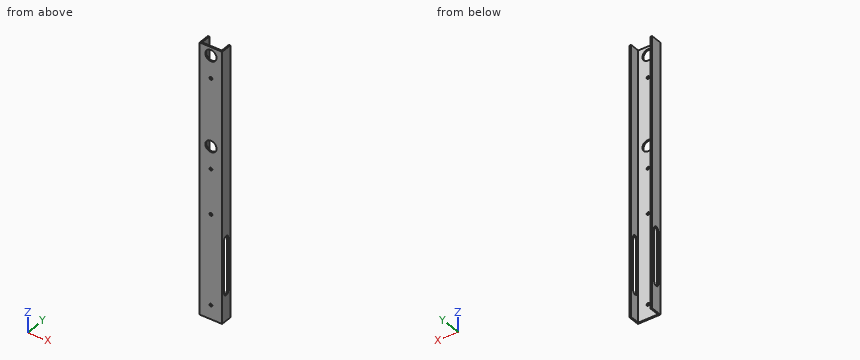
from build123d import *

# Parameters (mm, degrees)
BOSS_EXTRUDE1_DEPTH = 609.6
CUT_EXTRUDE1_REACH  = 5.175
SKETCH2_R           = 12.7
SKETCH2_R_2         = 3.175
CUT_EXTRUDE2_REACH  = 5.175
SKETCH3_R           = 3.175
CUT_EXTRUDE3_DEPTH  = 51.8


with BuildPart() as part:
    # Sketch1 → Boss-Extrude1 (new body)
    with BuildSketch(Plane.XY):
        Polygon((47.625, 3.175), (47.625, 25.4), (50.8, 25.4), (50.8, 0), (0, 0), (0, 25.4), (3.175, 25.4), (3.175, 3.175), align=None)
    extrude(amount=BOSS_EXTRUDE1_DEPTH)

    # Sketch2 → Cut-Extrude1 (cut, up to next)
    with BuildSketch(Plane(origin=(0, 3.175, 0), x_dir=(1, 0, 0), z_dir=(0, 1, 0)), mode=Mode.PRIVATE) as cut_extrude1_sk1:
        with Locations((25.4, -590.55)):
            Circle(SKETCH2_R)
    cut_extrude1_tool1 = extrude(cut_extrude1_sk1.sketch, amount=-CUT_EXTRUDE1_REACH, mode=Mode.PRIVATE) & part.part
    add(cut_extrude1_tool1.solids().sort_by_distance((25.4, 3.175, 590.55))[0], mode=Mode.SUBTRACT)
    # Sketch2 → Cut-Extrude1 (cut, up to next)
    with BuildSketch(Plane(origin=(0, 3.175, 0), x_dir=(1, 0, 0), z_dir=(0, 1, 0)), mode=Mode.PRIVATE) as cut_extrude1_sk2:
        with Locations((25.4, -387.35)):
            Circle(SKETCH2_R)
    cut_extrude1_tool2 = extrude(cut_extrude1_sk2.sketch, amount=-CUT_EXTRUDE1_REACH, mode=Mode.PRIVATE) & part.part
    add(cut_extrude1_tool2.solids().sort_by_distance((25.4, 3.175, 387.35))[0], mode=Mode.SUBTRACT)
    # Sketch2 → Cut-Extrude1 (cut, up to next)
    with BuildSketch(Plane(origin=(0, 3.175, 0), x_dir=(1, 0, 0), z_dir=(0, 1, 0)), mode=Mode.PRIVATE) as cut_extrude1_sk3:
        with Locations((25.4, -539.75)):
            Circle(SKETCH2_R_2)
    cut_extrude1_tool3 = extrude(cut_extrude1_sk3.sketch, amount=-CUT_EXTRUDE1_REACH, mode=Mode.PRIVATE) & part.part
    add(cut_extrude1_tool3.solids().sort_by_distance((25.4, 3.175, 539.75))[0], mode=Mode.SUBTRACT)
    # Sketch2 → Cut-Extrude1 (cut, up to next)
    with BuildSketch(Plane(origin=(0, 3.175, 0), x_dir=(1, 0, 0), z_dir=(0, 1, 0)), mode=Mode.PRIVATE) as cut_extrude1_sk4:
        with Locations((25.4, -336.55)):
            Circle(SKETCH2_R_2)
    cut_extrude1_tool4 = extrude(cut_extrude1_sk4.sketch, amount=-CUT_EXTRUDE1_REACH, mode=Mode.PRIVATE) & part.part
    add(cut_extrude1_tool4.solids().sort_by_distance((25.4, 3.175, 336.55))[0], mode=Mode.SUBTRACT)

    # Sketch3 → Cut-Extrude2 (cut, up to next)
    with BuildSketch(Plane(origin=(0, 3.175, 0), x_dir=(1, 0, 0), z_dir=(0, 1, 0)), mode=Mode.PRIVATE) as cut_extrude2_sk1:
        with Locations((25.4, -234.95)):
            Circle(SKETCH3_R)
    cut_extrude2_tool1 = extrude(cut_extrude2_sk1.sketch, amount=-CUT_EXTRUDE2_REACH, mode=Mode.PRIVATE) & part.part
    add(cut_extrude2_tool1.solids().sort_by_distance((25.4, 3.175, 234.95))[0], mode=Mode.SUBTRACT)
    # Sketch3 → Cut-Extrude2 (cut, up to next)
    with BuildSketch(Plane(origin=(0, 3.175, 0), x_dir=(1, 0, 0), z_dir=(0, 1, 0)), mode=Mode.PRIVATE) as cut_extrude2_sk2:
        with Locations((25.4, -31.75)):
            Circle(SKETCH3_R)
    cut_extrude2_tool2 = extrude(cut_extrude2_sk2.sketch, amount=-CUT_EXTRUDE2_REACH, mode=Mode.PRIVATE) & part.part
    add(cut_extrude2_tool2.solids().sort_by_distance((25.4, 3.175, 31.75))[0], mode=Mode.SUBTRACT)

    # Sketch4 → Cut-Extrude3 (cut, through all)
    with BuildSketch(Plane(origin=(50.8, 0, 0), x_dir=(0, 0, -1), z_dir=(1, 0, 0))):
        with BuildLine():
            Line((-183.606708986, 19.05), (-63.5, 19.05))
            ThreePointArc((-63.5, 19.05), (-57.15, 12.7), (-63.5, 6.35))
            Line((-63.5, 6.35), (-183.606708986, 6.35))
            ThreePointArc((-183.606708986, 6.35), (-189.956708986, 12.7), (-183.606708986, 19.05))
        make_face()
    extrude(amount=-CUT_EXTRUDE3_DEPTH, mode=Mode.SUBTRACT)


solid = part.part
The model under review builds one solid part; all positions refer to its coordinate system, in mm. Give positions to 0.01 mm unless a question says otherwise; leave off trailing zeros. Loops run counter-clockwise (first coordinate to the right, second up) from the corner with the lowest first, then second, coordinate; pieces in that order, holes last. Notation, with made-up numbers: (-5, 77) -> (44, 77) arc R25 ccw to (44, 94) -> close; hole circle Ø2 at (-7.75, 23.5). An arc over 180 degrees is marked (long way). Put each result on its own line as item: value. Start each with the question number.
1. We need section B-B on z = 387.35. State the section outline as (x, y) points (3 decimals), then the cut area to 3 significant figures.
2. We need section C-C on z = 197.5. State the section outline as (x, y) points (3 decimals).
3. Wall thickness on probe 1 along X at (y, z) = (0.7, 234.95) (3 decimals); probe 2 along X at (y, z) = (20, 124.5) (3 decimals); probe 3 along Y at (x, z) = (38, 169.5) (3 decimals): over which ranges is each line inside the solid? List them lowest first.
4. Clearance check with a flat-ended pin moving along its axis: P1, Ø8.5, axis at x = 25.4, z = 31.75, coming from the +Y side (3 decimals). State where the tip first meets the part, or that it passes through.
5. We need section A-A on y = 12.7. State the section outline as (x, z) points (3 decimals), then the cut area to 3 significant figures.
Determined:
1. outline: (0, 0) -> (12.7, 0) -> (12.7, 3.175) -> (3.175, 3.175) -> (3.175, 25.4) -> (0, 25.4) -> close; (38.1, 0) -> (50.8, 0) -> (50.8, 25.4) -> (47.625, 25.4) -> (47.625, 3.175) -> (38.1, 3.175) -> close
1. area: 222 mm^2
2. outline: (0, 0) -> (50.8, 0) -> (50.8, 25.4) -> (47.625, 25.4) -> (47.625, 3.175) -> (3.175, 3.175) -> (3.175, 25.4) -> (0, 25.4) -> close
3. probe 1: 0 to 22.225, 28.575 to 50.8
3. probe 2: 0 to 3.175, 47.625 to 50.8
3. probe 3: 0 to 3.175
4. P1: y = 3.175
5. outline: (0, 0) -> (3.175, 0) -> (3.175, 57.15) -> (0, 57.15) -> close; (0, 189.957) -> (3.175, 189.957) -> (3.175, 609.6) -> (0, 609.6) -> close; (47.625, 0) -> (50.8, 0) -> (50.8, 57.15) -> (47.625, 57.15) -> close; (47.625, 189.957) -> (50.8, 189.957) -> (50.8, 609.6) -> (47.625, 609.6) -> close
5. area: 3,030 mm^2
